Design review of the part shown in the three views and the two pictorial views. Dimensions are in mm from the part's minimum x, y and z. Coordinates: 2 decimals unless noted, no trailing zeros. Write each loop counter-clockwise with the first axis right and the second up, starting at its lowest first coordinate (ties: lowest second). Pieces come first, ordered by that corner, then holes.
Q1. Take a section at A-A, the plane z = 65. Write out the cut boundary in (x, y), plus the area to 4 significant figures.
Q2. Take a section at B-B, the plane y = 60. Write out the cut boundary in (x, z).
Q3. The part is to be moulded in two halves that separate along Z. For the marked faces 1, 2, 3 and 4, say which applies: released by +Z, released by -Z, zero draft, split by the parting line, or undercut.
Q4. Take a section at D-D, the plane y = 144. Write out the cut boundary in (x, z).
Q5. Take a section at C-C, the plane x = 27. Write out the cut boundary in (y, z), plus the area to 3 significant figures.
Q6. For L1, parallel to Z at x = 32.5, y = 72.5; L2, parallel to Z at x = 37.85, y = 60; L3, parallel to X at y = 165, z = 37, list the stretches that pass through material, from the lowest coordinate up.
Q7. For pin 1 Ø2 at (y, z) = (79, 115.5) entering from -X, flat-tipped, find the tip position at first contact; note if it passes through.
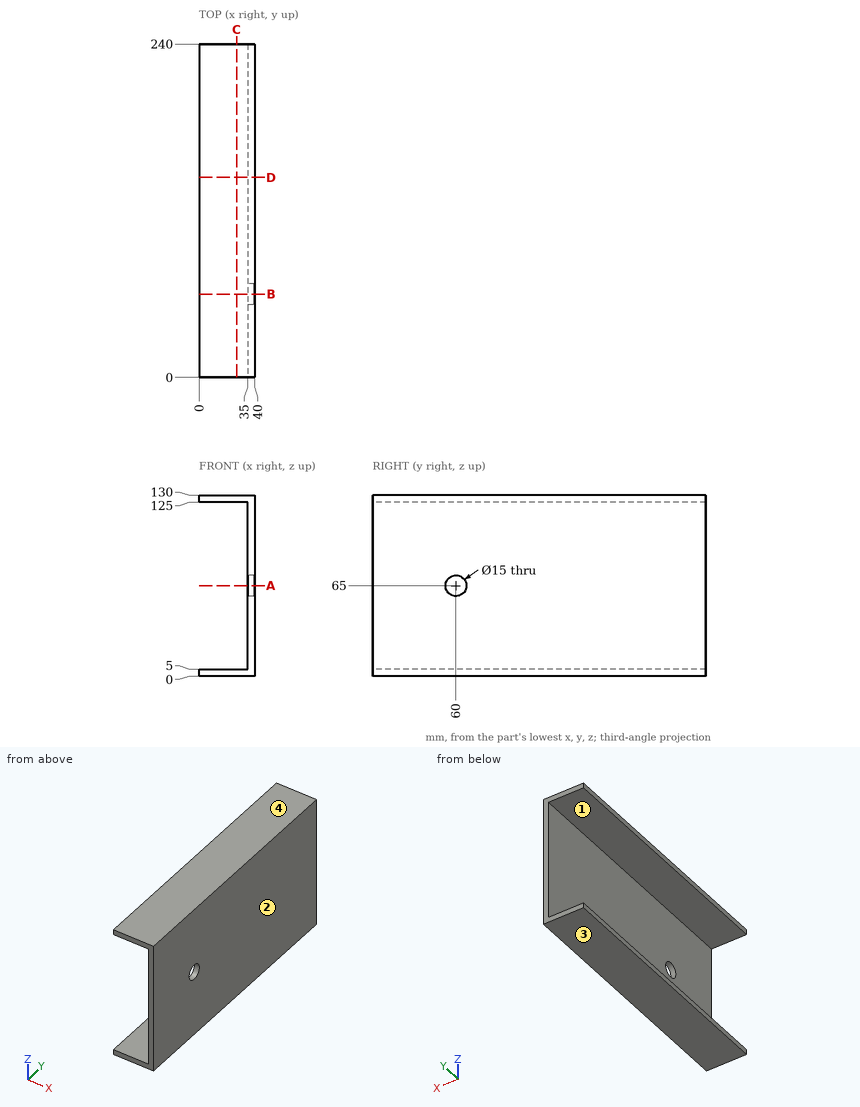
Responses:
1. outline: (35, 0) - (40, 0) - (40, 52.5) - (35, 52.5) - close; (35, 67.5) - (40, 67.5) - (40, 240) - (35, 240) - close
1. area: 1,125 mm2
2. outline: (0, 0) - (40, 0) - (40, 57.5) - (35, 57.5) - (35, 5) - (0, 5) - close; (0, 125) - (35, 125) - (35, 72.5) - (40, 72.5) - (40, 130) - (0, 130) - close
3. face 1: undercut
3. face 2: zero draft
3. face 3: released by -Z
3. face 4: released by +Z
4. outline: (0, 0) - (40, 0) - (40, 130) - (0, 130) - (0, 125) - (35, 125) - (35, 5) - (0, 5) - close
5. outline: (0, 0) - (240, 0) - (240, 5) - (0, 5) - close; (0, 125) - (240, 125) - (240, 130) - (0, 130) - close
5. area: 2,400 mm2
6. L1: z = 0 to 5, 125 to 130
6. L2: z = 0 to 57.5, 72.5 to 130
6. L3: x = 35 to 40
7. pin 1: stops at x = 35
